```python
from build123d import *

# Parameters (mm, degrees)
F2_DEPTH     = 6.604
F4_W         = 17.018
F4_H         = 5.5950877881
F5_DEPTH     = 71.6798
F6_W         = 16.355678454
F6_H         = 4.3095059386
F7_DEPTH     = 44.9793598678
F9_DEPTH     = 56.897
F10_W        = 342.8717973226
F10_H        = 3.7084
F11_DEPTH    = 1.27
F12_T1_DEPTH = 3.7084
F14_DEPTH    = 4.065


# Not quite as in the source:
# - a fillet or chamfer that OpenCascade refuses, or shapes differently, is made with other operations: its cross-section is extruded or revolved along the edge and cut away or added


with BuildPart() as f2:
    # F1 (on Top) → F2 (new body)
    with BuildSketch(Plane.XY):
        Polygon((80.7733850724, 0), (80.7733850724, 24.9428), (15.7493850724, 24.9428), (15.7493850724, 30.8864), (16.6319306082, 31.5163598678), (16.6319306082, 44.9783598678), (13.1174201358, 42.4697068149), (9.0945850724, 28.2448), (9.0945850724, 8.9408), (24.4869850724, 8.9408), (24.4869850724, -11.8872), (23.8773850724, -13.1876401322), (23.8773850724, -57.1296401322), (31.1824725433, -53.0194550947), (38.2029850724, -10.414), (38.2029850724, 0), align=None)
    extrude(amount=F2_DEPTH)

    # F4 (on face) → F5 (cut, through all)
    with BuildSketch(Plane(origin=(9.0945850724, 0, 0), x_dir=(0, -1, 0), z_dir=(-1, 0, 0))):
        with Locations((-12.4714, 5.3375438941)):
            Rectangle(F4_W, F4_H)
    extrude(amount=-F5_DEPTH, mode=Mode.SUBTRACT)

    # F6 (on Front) → F7 (cut, through all)
    with BuildSketch(Plane.XZ):
        with Locations((16.3091458454, 4.6947529693)):
            Rectangle(F6_W, F6_H)
    extrude(amount=-F7_DEPTH, mode=Mode.SUBTRACT)

    # F8 (on face) → F9 (cut, through all)
    with BuildSketch(Plane(origin=(23.8773850724, 0, 0), x_dir=(0, -1, 0), z_dir=(-1, 0, 0))):
        Polygon((57.1296401322, -1.4798081247), (57.1296401322, 2.794), (2.9003161471, 2.794), (2.032, -1.4798081247), align=None)
    extrude(amount=-F9_DEPTH, mode=Mode.SUBTRACT)

    # F10 (on face) → F11 (join)
    with BuildSketch(Plane.XY.offset(2.54)):
        with Locations((237.7086864111, 12.4714)):
            Rectangle(F10_W, F10_H)
    extrude(amount=F11_DEPTH)

    # F12: fillet of radius 6.35 on 1 edges, made by hand

    # F12_s2 → F12_t1 (cut)
    with BuildSketch(Plane.XZ.offset(-14.3256)):
        with BuildLine():
            ThreePointArc((66.2727877498, 2.54), (68.0747414356, 3.4841389426), (70.0827877498, 3.81))
            Line((70.0827877498, 3.81), (66.2727877498, 3.81))
            Line((66.2727877498, 3.81), (66.2727877498, 2.54))
        make_face()
    extrude(amount=F12_T1_DEPTH, mode=Mode.SUBTRACT)

    # F13 (on face) → F14 (cut, through all)
    with BuildSketch(Plane(origin=(0, 0, 2.54), x_dir=(1, 0, 0), z_dir=(0, 0, -1))):
        with BuildLine():
            ThreePointArc((403.4869184795, -12.5476), (402.7459176611, -12.8545325887), (402.4389850724, -13.5955334071))
            Line((402.4389850724, -13.5955334071), (402.4389850724, -14.3256))
            Line((402.4389850724, -14.3256), (409.480124712, -15.0942075998))
            Line((409.480124712, -15.0942075998), (409.1445850724, -12.5476))
            Line((409.1445850724, -12.5476), (403.4869184795, -12.5476))
        make_face()
    extrude(amount=-F14_DEPTH, mode=Mode.SUBTRACT)


solid = f2.part
```
Can you work these out from the model? Positions are in its coordinate system, mm. A direction names the side the tool comes from. Give positions to 0.01 mm unless a question says otherwise; leave off trailing zeros. Order: outer loops, then holes, each group sorted by start corner. A loop starts at its lowest first (then second) coordinate and runs counter-clockwise, first axis right, second up. Notation, with made-up numbers: (41.25, 75) - (70.25, 75) arc R30 ccw to (70.25, 101) - close; hole circle Ø11 at (27, 32.25). An arc over 180 degrees is marked (long way). Use a Markdown table: item, result. Add a question column.
Q1. If we mould it in two halves opening along Y, with no side actions, what happens to faces 5 (the flat face through (34.644, -32.015, 4.672)), 6 (the flat face through (44, 11, 0)), 7 (the flat face through (36, 16, 2.54))? For each: released by +Y, released by -Y, zero draft, split by the parting line, or undercut.
Q2. On a 3-axis mill with a long thin cutter (end or side, diameter ignored), from which of +Z, -Z, +X, -X, +Y, -Y can I reach the whole of each face in a straight line? I mean faces 1 (the flat face through (35, -17, 6.604)), 2 (the flat face through (38.203, -4, 4)), 3 (the flat face through (24.487, -1, 3)), 4 (the flat face through (29, -24, 2.794)). Say none if no direction works.
Q3. If we section it at A-A on x = 358.5: Write out the boundary of the cut face in (y, z), plus the area to 3 significant figures.
Q4. I'm going to push flat-ended pins straight in: pin 1 (6 mm diameter, centred on x = 180.5, y = 20, fed in from -Z); pin 2 (3 mm diameter, centred on y = 26.5, z = 0.5, fed in from +X); pin 3 (4 mm diameter, centred on x = 212, y = 12.5, fed in from -Z); pin 4 (4.5 mm diameter, centred on x = 30, y = -33, fed in from -Z). Where does each tip first touch, or does it pass through?
Q5. Please list where these lines run through material, in increasing order: line 1 along Y through (x, z) = (77.5, 4); line 2 along X through (y, z) = (27.5, 2.5); line 3 along Y through (x, z) = (67, 1.5).
Q6. If we section it at B-B on y = -24.5: Write out the boundary of the cut face in (x, z), plus the area to 3 significant figures.
Answers follow:
| question | item | result |
|---|---|---|
| 1 | face 5 | released by -Y |
| 1 | face 6 | zero draft |
| 1 | face 7 | undercut |
| 2 | face 1 | +Z, +X, -X, +Y, -Y |
| 2 | face 2 | +Z, -Z, +X, -Y |
| 2 | face 3 | +Z, -Z, -X |
| 2 | face 4 | -Z, +X, -X, -Y |
| 3 | outline | (10.62, 2.54) - (14.33, 2.54) - (14.33, 3.81) - (10.62, 3.81) - close |
| 3 | area | 4.71 mm^2 |
| 4 | pin 1 | passes through |
| 4 | pin 2 | stops at x = 15.75 |
| 4 | pin 3 | stops at z = 2.54 |
| 4 | pin 4 | stops at z = 2.79 |
| 5 | line 1 | y = 0 to 3.96, 20.98 to 24.94 |
| 5 | line 2 | x = 9.09 to 15.75 |
| 5 | line 3 | y = 0 to 24.94 |
| 6 | outline | (23.88, 2.79) - (35.88, 2.79) - (35.88, 6.6) - (23.88, 6.6) - close |
| 6 | area | 45.7 mm^2 |
